Design review of the part built by this model. Coordinates are the model's own, in mm. A direction names the side the tool comes from. Give positions to 0.01 mm unless a question says otherwise; leave off trailing zeros. Loops run counter-clockwise (first coordinate to the right, second up) from the corner with the lowest first, then second, coordinate; pieces in that order, holes last. Notation, with made-up numbers: M 88.5,-2 L 105.5,-2 A24 cw 105.5,13 Z; hole C 33.25,63.5 d11. An arc over 180 degrees is marked long. Use a Markdown table: item, result. Add a question column.
(1) Add section A-A, the plane y = 70.5. Give the boundary of the cut face in (x, z).
(2) Add section C-C, the plane x = 6. Give the boundary of the cut face in (y, z), then the cut area to 3 significant figures.
(3) Insertion check: pin 1 Ø1 at (x, z) = (41.5, 1) entering from +Y; pin 2 Ø3 at (x, y) = (67.05, 21.79) entering from -Z; pin 3 Ø8 at (x, y) = (51.5, 14) entering from -Z; pin 4 Ø1 at (x, z) = (-43.5, 4.5) entering from +Y. Each pin has a flat end and moves straight along its axis. Give the tip position at first contact, or say it passes through.
(4) Add section D-D, the plane y = 0. Give the boundary of the cut face in (x, z), then the cut area to 3 significant figures.
(5) For probe 1 along X at (y, z) = (20.5, 0.45); probe 2 along X at (y, z) = (72.5, 2.4); probe 3 along Y at (x, z) = (65, 2.4), list the stretches that pass through material, from the lowest coordinate up.
(6) Draft analysis for pull direction X (two halves, no side actions). For faces 1 (the face through (54.39, 7.7, 0.99)), 2 (the face through (64.3, 21.9, 3.7)), 3 (the face through (26, -41.707, 3)), state which applies: pulls with the +X half, pulls with the -X half, needs draft (parallel to the pull), parting line crosses it, or undercut.
(7) For faces 4 (the face through (-69.797, 21.907, 3.725)), 5 (the face through (-9.22, 54.92, 0.99)), 6 (the face through (36.955, -26.237, 3.726)), 7 (the face through (5.622, -37.507, 3.726)), list the 3-axis set-ups (+Z, -Z, +X, -X, +Y, -Y) from which the entire face can be reached by the end or side of a thin tool; tool diameter is ignored.
(8) Add section B-B, the plane z = 4.05. Give the boundary of the cut face in (x, y).
```python
from build123d import *

# Parameters (mm, degrees)
SALIENTE_EXTRUIR1_DEPTH = 2
SALIENTE_EXTRUIR2_DEPTH = 3.5
CROQUIS2_R              = 1.85
CORTAR_EXTRUIR4_DEPTH   = 10
CROQUIS4_R              = 2.75
CORTAR_EXTRUIR5_DEPTH   = 3.6


with BuildPart() as part:
    # Croquis1 → Saliente-Extruir1 (new body)
    with BuildSketch(Plane.XY):
        Polygon((79.216456577, 25.738987008), (18.700468689, 25.738987008), (0, 83.293111629), (-18.700468689, 25.738987008), (-79.216456577, 25.738987008), (-30.257993944, -9.831418201), (-40.615003785, -41.707016882), (-13.615003785, -41.707016882), (0, -31.815137614), (13.615003785, -41.707016882), (40.615003785, -41.707016882), (30.257993944, -9.831418201), align=None)
    extrude(amount=SALIENTE_EXTRUIR1_DEPTH)

    # Croquis3 → Saliente-Extruir2 (add)
    with BuildSketch(Plane.XY.offset(2)):
        Polygon((-41.981904677, -41.707016882), (-11.403311683, -41.707016882), (0, -33.422025984), (11.403311683, -41.707016882), (41.981904677, -41.707016882), (31.7862356, -10.327974016), (83.217445176, 27.038987008), (19.644973975, 27.038987008), (0, 87.5), (-19.644973975, 27.038987008), (-83.217445176, 27.038987008), (-31.7862356, -10.327974016), align=None)
    extrude(amount=SALIENTE_EXTRUIR2_DEPTH)

    # Croquis2 → Cortar-Extruir4 (cut)
    with BuildSketch(Plane.XY.offset(5.5)):
        with Locations((0, 70.5)):
            Circle(CROQUIS2_R)
        with Locations((67.049484399, 21.785698103)):
            Circle(CROQUIS2_R)
        with Locations((-67.049484399, 21.785698103)):
            Circle(CROQUIS2_R)
    extrude(amount=-CORTAR_EXTRUIR4_DEPTH, mode=Mode.SUBTRACT)

    # Croquis4 → Cortar-Extruir5 (cut)
    with BuildSketch(Plane.XY.offset(5.5)):
        with Locations((67.049484399, 21.785698103)):
            Circle(CROQUIS4_R)
        with Locations((0, 70.5)):
            Circle(CROQUIS4_R)
        with Locations((-67.049484399, 21.785698103)):
            Circle(CROQUIS4_R)
    extrude(amount=-CORTAR_EXTRUIR5_DEPTH, mode=Mode.SUBTRACT)


solid = part.part
```
Established:
| question | item | result |
|---|---|---|
| 1 | outline | M -5.52,2 L -4.16,2 L -4.16,0 L -1.85,0 L -1.85,1.9 L -2.75,1.9 L -2.75,5.5 L -5.52,5.5 Z; M 1.85,0 L 4.16,0 L 4.16,2 L 5.52,2 L 5.52,5.5 L 2.75,5.5 L 2.75,1.9 L 1.85,1.9 Z |
| 2 | outline | M -37.78,2 L -36.17,2 L -36.17,0 L 64.83,0 L 64.83,2 L 69.03,2 L 69.03,5.5 L -37.78,5.5 Z |
| 2 | area | 576 mm^2 |
| 3 | pin 1 | y = 25.74 |
| 3 | pin 2 | through |
| 3 | pin 3 | z = 0 |
| 3 | pin 4 | y = 27.04 |
| 4 | outline | M -46,2 L -43.79,2 L -43.79,0 L 43.79,0 L 43.79,2 L 46,2 L 46,5.5 L -46,5.5 Z |
| 4 | area | 497 mm^2 |
| 5 | probe 1 | -72.01 to -68.38, -65.72 to 65.72, 68.38 to 72.01 |
| 5 | probe 2 | -4.87 to -1.89, 1.89 to 4.87 |
| 5 | probe 3 | 13.8 to 19.95, 23.62 to 27.04 |
| 6 | face 1 | pulls with the +X half |
| 6 | face 2 | undercut |
| 6 | face 3 | needs draft |
| 7 | face 4 | +Z |
| 7 | face 5 | -Z, -X, +Y |
| 7 | face 6 | +Z, -Z, +X |
| 7 | face 7 | +Z, -Z, -Y |
| 8 | outline | M -83.22,27.04 L -31.79,-10.33 L -41.98,-41.71 L -11.4,-41.71 L 0,-33.42 L 11.4,-41.71 L 41.98,-41.71 L 31.79,-10.33 L 83.22,27.04 L 19.64,27.04 L 0,87.5 L -19.64,27.04 Z; hole C -67.05,21.79 d5.5; hole C 0,70.5 d5.5; hole C 67.05,21.79 d5.5 |
